Can you work these out from the model? Positions are in its coordinate system, mm. Coordinates: 2 decimals unless noted, no trailing zeros. Loops run counter-clockwise (first coordinate to the right, second up) from the corner with the lowest first, then second, coordinate; pieces in that order, holes last. Notation, with made-up numbers: M 19,20.25 L 40,20.25 A11 cw 40,36.25 Z; hole C 41.25,29 d9. An arc over 180 degrees is marked long. Answer as a JSON object with one key per item and string values. Group by question number.
Item 1: We'd pull the mould along Z, two halves only. Please class faces 1 (the flat face through (-18, 5, -4)), 2 (the flat face through (-18, 0, -4)): +Z half, -Z half, draft (parallel to the pull), parting line (faces both ways), or undercut.
Item 2: Suppose I cut it at A-A (y = -1.5). Count the separate pieces of the cut face and the enclosed holes in it, then the cut area to 3 significant figures.
Item 3: Suppose I cut it at D-D (x = -31). Write out the boundary of the cut face in (y, z), then the cut area to 3 significant figures.
Item 4: I'm going to push a flat-ended pin straight in: pin 1 Ø3 at (x, z) = (-18.5, -3.5) entering from -Y. Where does the tip first touch, or does it pass through?
Item 5: If I drill on line 1 (Y direction, x = -14, z = -5.5); line 2 (Z direction, x = -20.5, y = 1.75); line 3 (Y direction, x = -34.5, z = -9), over which ranges is the centre line in solid material (lowest first)?
Autodesk Inventor part; units mm, degrees
ref_plane "YZ Plane" through (0, 0, 0) normal (1, 0, 0) x (0, 1, 0)
ref_plane "XZ Plane" through (0, 0, 0) normal (0, 1, 0) x (-1, 0, 0)
ref_plane "XY Plane" through (0, 0, 0) normal (0, 0, 1) x (1, 0, 0)
sketch "Sketch1" plane through (0, 0, 0) normal (0, 1, 0) x (-1, 0, 0)
  line L0 (0, 0) -> (37, 0)
  line L1 (37, -7.5) -> (0, -7.5)
  line L2 (0, -7.5) -> (0, 0)
  arc A0 (37, -2.75) -> (37, -4.75) centre (37, -3.75) ccw
  line L3 (37, 0) -> (37, -2.75)
  line L4 (37, -4.75) -> (37, -7.5)
  dimension "d0" = 37
  dimension "d1" = 7.5
  dimension "d2" = 2
extrude "Extrusion1" add sketch "Sketch1" along normal blind 5
sketch "Sketch2" plane through (-37, 0, 0) normal (0, 0, 1) x (1, 0, 0)
  circle A0 centre (2.5, 2.5) radius 0.3
  circle A1 centre (5, 2.5) radius 0.3
  circle A2 centre (7.5, 2.5) radius 0.3
  circle A3 centre (10, 2.5) radius 0.3
  circle A4 centre (12.5, 2.5) radius 0.3
  circle A5 centre (15, 2.5) radius 0.3
  circle A6 centre (17.5, 2.5) radius 0.3
  circle A7 centre (20, 2.5) radius 0.3
  circle A8 centre (22.5, 2.5) radius 0.3
  circle A9 centre (25, 2.5) radius 0.3
  circle A10 centre (27.5, 2.5) radius 0.3
  circle A11 centre (30, 2.5) radius 0.3
  circle A12 centre (32.5, 2.5) radius 0.3
  circle A13 centre (35, 2.5) radius 0.3
  point P0 (37, 0)
  dimension "d5" = 0.6
  dimension "d7" = 0.6
  dimension "d8" = 0.6
  dimension "d9" = 0.6
  dimension "d11" = 0.6
  dimension "d12" = 0.6
  dimension "d13" = 0.6
  dimension "d14" = 0.6
  dimension "d15" = 0.6
  dimension "d16" = 0.6
  dimension "d17" = 0.6
  dimension "d18" = 0.6
  dimension "d19" = 0.6
  dimension "d20" = 0.6
sketch3d "3D Sketch1"
  line L0 (-2, 2.5, 0) -> (-2, 2.5, 2)
  line L1 (-2, 2.5, 2) -> (-2, -5, 2)
  dimension "d23" = 2
  dimension "d24" = 7.5
sweep "Sweep1" add profiles "Sketch2" path "3D Sketch1"
sketch "Sketch3" plane through (0, 0, -7.5) normal (0, 0, -1) x (-1, 0, 0)
  arc A0 (2.3, 2.5) -> (1.7, 2.5) centre (2, 2.5) ccw
  circle A1 centre (2, 2.5) radius 0.3
  arc A2 (4.8, 2.5) -> (4.2, 2.5) centre (4.5, 2.5) ccw
  circle A3 centre (4.5, 2.5) radius 0.3
  circle A4 centre (7, 2.5) radius 0.3
  circle A5 centre (7, 2.5) radius 0.3
  circle A6 centre (9.5, 2.5) radius 0.3
  circle A7 centre (9.5, 2.5) radius 0.3
  circle A8 centre (12, 2.5) radius 0.3
  circle A9 centre (12, 2.5) radius 0.3
  arc A10 (14.2, 2.5) -> (14.8, 2.5) centre (14.5, 2.5) ccw
  circle A11 centre (14.5, 2.5) radius 0.3
  circle A12 centre (17, 2.5) radius 0.3
  circle A13 centre (17, 2.5) radius 0.3
  circle A14 centre (19.5, 2.5) radius 0.3
  circle A15 centre (19.5, 2.5) radius 0.3
  circle A16 centre (22, 2.5) radius 0.3
  circle A17 centre (22, 2.5) radius 0.3
  circle A18 centre (24.5, 2.5) radius 0.3
  circle A19 centre (24.5, 2.5) radius 0.3
  circle A20 centre (29.5, 2.5) radius 0.3
  circle A21 centre (29.5, 2.5) radius 0.3
  circle A22 centre (27, 2.5) radius 0.3
  circle A23 centre (27, 2.5) radius 0.3
  circle A24 centre (32, 2.5) radius 0.3
  circle A25 centre (32, 2.5) radius 0.3
  circle A26 centre (34.5, 2.5) radius 0.3
  circle A27 centre (34.5, 2.5) radius 0.3
  point P0 (0, 0)
sketch3d "3D Sketch2"
  line L0 (-2, 2.5, -7.5) -> (-2, 2.5, -9.5)
  line L1 (-2, 2.5, -9.5) -> (-2, -5, -9.5)
  dimension "d27" = 2
  dimension "d28" = 7.5
sweep "Sweep2" add profiles "Sketch3" path "3D Sketch2"
equation "\"BendRadius\" = Thickness"
equation "\"BendReliefWidth\" = Thickness"
equation "\"BendReliefDepth\" = 0.5 * Thickness"
equation "\"CornerReliefSize\" = 4 * Thickness"
equation "\"MinimumRemnant\" = 2 * Thickness"
equation "\"TransitionRadius\" = BendRadius"
equation "\"JacobiRadiusSize\" = BendRadius"
equation "\"GapSize\" = Thickness"
From the geometry:
{
 "1": {"face 1": "draft", "face 2": "undercut"},
 "2": {"separate pieces": "28", "enclosed holes": "0", "area": "7.92 mm2"},
 "3": {"outline": "M 0,-7.5 L 5,-7.5 L 5,0 L 0,0 Z", "area": "37.5 mm2"},
 "4": {"pin 1": "y = 0"},
 "5": {"line 1": "0 to 5", "line 2": "-7.5 to 0", "line 3": "2.2 to 2.8"}
}
